```python
from build123d import *

# Parameters (mm, degrees)
EXTRUDE_1_DEPTH     = 2
SKETCH_2_W          = 4
SKETCH_2_H          = 5
EXTRUDE_2_DEPTH     = 15
SKETCH_3_R          = 1.05
CUT_EXTRUDE_1_DEPTH = 12
SKETCH_5_R          = 1.75
CUT_EXTRUDE_2_DEPTH = 12
FILLET_1_R          = 1
FILLET_2_R          = 1


with BuildPart() as part:
    # 草图1 → 凸台-拉伸1 (new body)
    with BuildSketch(Plane(origin=(0, 0, 0), x_dir=(1, 0, 0), z_dir=(0, 1, 0))):
        Polygon((0, -5), (13, -5), (16, -5), (16, 0), (13, 0), (0, 0), (-3, 0), (-3, -5), align=None)
    extrude(amount=EXTRUDE_1_DEPTH)

    # 草图2 → 凸台-拉伸2 (add)
    with BuildSketch(Plane(origin=(0, 2, 0), x_dir=(1, 0, 0), z_dir=(0, 1, 0))):
        with Locations((6.5, -2.5)):
            Rectangle(SKETCH_2_W, SKETCH_2_H)
    extrude(amount=EXTRUDE_2_DEPTH)

    # 草图3 → 切除-拉伸1 (cut)
    with BuildSketch(Plane.ZY.offset(-4.5)):
        with Locations((2.5, 15)):
            Circle(SKETCH_3_R)
        with Locations((2.5, 6)):
            Circle(SKETCH_3_R)
    extrude(amount=-CUT_EXTRUDE_1_DEPTH, mode=Mode.SUBTRACT)

    # 草图5 → 切除-拉伸2 (cut)
    with BuildSketch(Plane(origin=(0, 2, 0), x_dir=(1, 0, 0), z_dir=(0, 1, 0))):
        with Locations(Location((0, -2.5, 0), (0, 0, 270))):
            Circle(SKETCH_5_R)
        with Locations(Location((13, -2.5, 0), (0, 0, 270))):
            Circle(SKETCH_5_R)
    extrude(amount=-CUT_EXTRUDE_2_DEPTH, mode=Mode.SUBTRACT)

    # 圆角1
    fillet_1_edges = [part.edges().sort_by_distance(p)[0] for p in [
        (16, 1, 0),
        (16, 1, 5),
        (-3, 1, 5),
        (-3, 1, 0),
    ]]
    fillet(fillet_1_edges, radius=FILLET_1_R)

    # 圆角2
    fillet_2_edges = [part.edges().sort_by_distance(p)[0] for p in [
        (6.5, 17, 0),
        (6.5, 17, 5),
    ]]
    fillet(fillet_2_edges, radius=FILLET_2_R)


solid = part.part
```
Geometry check sheet. Reference: the model listing, model coordinates, mm. A direction names the side the tool comes from. Give positions to 0.01 mm unless a question says otherwise; leave off trailing zeros. Loops run counter-clockwise (first coordinate to the right, second up) from the corner with the lowest first, then second, coordinate; pieces in that order, holes last. Notation, with made-up numbers: M 62.5,62.5 L 77.5,62.5 A24 cw 77.5,83.5 Z; hole C 12.5,66 d8. An arc over 180 degrees is marked long. Answer as CSV lines item,"result".
Item 1: Cross-section at A-A on z = 2.5. Record the cut outline in (x, y), and give its area (3 significant figures).
Values:
outline,"M -3,0 L -1.75,0 L -1.75,2 L -3,2 Z; M 1.75,0 L 11.25,0 L 11.25,2 L 8.5,2 L 8.5,4.95 L 4.5,4.95 L 4.5,2 L 1.75,2 Z; M 4.5,7.05 L 8.5,7.05 L 8.5,13.95 L 4.5,13.95 Z; M 4.5,16.05 L 8.5,16.05 L 8.5,17 L 4.5,17 Z; M 14.75,0 L 16,0 L 16,2 L 14.75,2 Z"
area,"67.2 mm²"
Item 2: Cross-section at D-D on y = 6. Record the cut outline in (x, z), and give its area (3 significant figures).
Values:
outline,"M 4.5,0 L 8.5,0 L 8.5,1.45 L 4.5,1.45 Z; M 4.5,3.55 L 8.5,3.55 L 8.5,5 L 4.5,5 Z"
area,"11.6 mm²"
Item 3: Cross-section at C-C on x = 7. Record the cut outline in (y, z), and give its area (3 significant figures).
Values:
outline,"M 0,0 L 16,0 A1 ccw 17,1 L 17,4 A1 ccw 16,5 L 0,5 Z; hole C 6,2.5 d2.1; hole C 15,2.5 d2.1"
area,"77.6 mm²"
Item 4: Depth check by flat-ended pin: P1, Ø1.5, axis at x = -1, z = 3, coming from the +Y side; P2, Ø1, axis at y = 12.5, z = 2, coming from the -X side; P3, Ø1.5, axis at x = 10, y = 7.5, coming from the -Z side; P4, Ø1, axis at x = 10, z = 1, coming from the -Y side. Enter the tip coordinate at first touch or a pass-through.
Values:
P1,"stops at y = 2"
P2,"stops at x = 4.5"
P3,"passes through"
P4,"stops at y = 0"
Item 5: Access from +Z, -Z, +X, -X, +Y, -Y to the whole of each face (thin tool, end or side, straight path). Record for faces 5 (the cylindrical face through (6.528, 16.699, 4.715)), 6 (the flat face through (11, 2, 1)), 7 (the flat face through (4.5, 9, 3)).
Values:
face 5,"+Z, +X, -X, +Y"
face 6,"+Z, -Z, +X, +Y"
face 7,"+Z, -Z, -X, +Y"
Item 6: Material ranges on line 1 (Y direction, x = 6, z = 2.55); line 2 (X direction, y = 1, z = 2.8); line 3 (Y direction, x = 5.5, z = 2.95), recorded low to high.
Values:
line 1,"y = 0 to 4.95, 7.05 to 13.95, 16.05 to 17"
line 2,"x = -3 to -1.72, 1.72 to 11.28, 14.72 to 16"
line 3,"y = 0 to 5.05, 6.95 to 14.05, 15.95 to 17"
Item 7: Release check for a two-part mould opening along Y. For faces 1 (the flat face through (6, 17, 2)), 2 (the flat face through (6, 0, 2)), 3 (the cylindrical face through (6.47, 7.04, 2.36)), 4 (the flat face through (6, 6, 5)) record: pulls with the +Y half, pulls with the -Y half, needs draft (parallel to the pull), parting line crosses it, or undercut.
Values:
face 1,"pulls with the +Y half"
face 2,"pulls with the -Y half"
face 3,"undercut"
face 4,"needs draft"
Item 8: Cross-section at B-B on x = 13. Record the cut outline in (y, z).
Values:
outline,"M 0,0 L 2,0 L 2,0.75 L 0,0.75 Z; M 0,4.25 L 2,4.25 L 2,5 L 0,5 Z"
